from build123d import *

# Parameters (mm, degrees)
BOSS_EXTRU_1_DEPTH      = 30
ESQUISSE2_R             = 15
BOSS_EXTRU_2_DEPTH      = 5
BOSS_EXTRU_3_DEPTH      = 10
ESQUISSE7_R             = 2
ENL_V_MAT_EXTRU_1_DEPTH = 10


with BuildPart() as part:
    # Esquisse1 → Boss.-Extru.1 (new body)
    with BuildSketch(Plane.XY):
        Polygon((-14.849242405, 0), (0, 14.849242405), (14.849242405, 0), (19.849242405, 0), (0, 19.849242405), (-19.849242405, 0), align=None)
    extrude(amount=BOSS_EXTRU_1_DEPTH)

    # Esquisse2 → Boss.-Extru.2 (add)
    with BuildSketch(Plane(origin=(0, 14.849242405, 0), x_dir=(1, 0, 0), z_dir=(0, 1, 0))):
        with Locations((0, -15)):
            Circle(ESQUISSE2_R)
    extrude(amount=BOSS_EXTRU_2_DEPTH)

    # Esquisse5 → Boss.-Extru.3 (add)
    with BuildSketch(Plane(origin=(0, 19.849242405, 0), x_dir=(1, 0, 0), z_dir=(0, 1, 0))):
        with BuildLine():
            ThreePointArc((5, -9.409830056), (0, -7.5), (-5, -9.409830056))
            Line((-5, -9.409830056), (-5, -15))
            Line((-5, -15), (5, -15))
            Line((5, -15), (5, -9.409830056))
        make_face()
        with BuildLine():
            Line((5, -15), (-5, -15))
            Line((-5, -15), (-5, -20.590169944))
            ThreePointArc((-5, -20.590169944), (0, -22.5), (5, -20.590169944))
            Line((5, -20.590169944), (5, -15))
        make_face()
    extrude(amount=BOSS_EXTRU_3_DEPTH)

    # Esquisse7 → Enlèv. mat.-Extru.1 (cut)
    with BuildSketch(Plane.ZY.offset(5)):
        with Locations((15, 24.849242405)):
            Circle(ESQUISSE7_R)
    extrude(amount=-ENL_V_MAT_EXTRU_1_DEPTH, mode=Mode.SUBTRACT)


solid = part.part
Here's how the part is built. I have some questions about the finished solid (model axes, mm). A direction names the side the tool comes from. Give positions to 0.01 mm unless a question says otherwise; leave off trailing zeros. Order: outer loops, then holes, each group sorted by start corner. A loop starts at its lowest first (then second) coordinate and runs counter-clockwise, first axis right, second up. Notation, with made-up numbers: (-16, -29.75) -> (-6, -29.75) arc R20 ccw to (-6, 0.25) -> close; hole circle Ø5 at (15.25, 15.5). An arc over 180 degrees is marked (long way). Use a Markdown table: item, result. Add a question column.
Item 1: I need wall thicknesses on line 1 (Y direction, x = -13, z = 17.5); line 2 (Z direction, x = -2.5, y = 24.25); line 3 (X direction, y = 7.5, z = 17). Which ranges of each line are inside material? Lowest first, please.
Item 2: Imagine slicing it at D-D on x = 4. Please give me the cut outline in (y, z).
Item 3: Imagine slicing it at A-A on z = 15. Please give me the cut outline in (x, y).
Item 4: If we mould it in two halves opening along Y, with no side actions, what happens to faces 4 (the face through (0.1, 24.8, 7.5)), 5 (the face through (-11.99, 7.86, 14.79)), 6 (the face through (-17, 0, 15))? For each: pulls with the +Y half, pulls with the -Y half, needs draft (parallel to the pull), parting line crosses it, or undercut.
Item 5: Imagine slicing it at C-C on x = -5.5. Please give me the cut outline in (y, z).
Item 6: For faces 1 (the face through (-15, 17, 15)), 2 (the face through (5, 22.6, 15.1)), 3 (the face through (-5, 22.6, 14.9)), which set-ups out of +Z, -Z, +X, -X, +Y, -Y let a thin tool reach every point of the face, with its end or its side?
Item 7: Will these pins go through, and if not, where does the flat tip stop? pin 1 (5 mm diameter, centred on x = 0, y = 26, fed in from -Z); pin 2 (2 mm diameter, centred on y = 12, z = 20, fed in from -X); pin 3 (11 mm diameter, centred on x = 8, z = 9.5, fed in from -Y); pin 4 (2 mm diameter, centred on x = -6.5, y = 25.5, fed in from +Z).
Item 8: Imagine slicing it at B-B on y = 13. Please give me the cut outline in (x, z).
Data:
| question | item | result |
|---|---|---|
| 1 | line 1 | y = 1.85 to 6.85, 14.85 to 19.85 |
| 1 | line 2 | z = 7.93 to 13.09, 16.91 to 22.07 |
| 1 | line 3 | x = -12.35 to -7.35, 7.35 to 12.35 |
| 2 | outline | (10.85, 0) -> (15.85, 0) -> (15.85, 0.54) -> (19.85, 0.54) -> (19.85, 8.66) -> (29.85, 8.66) -> (29.85, 21.34) -> (19.85, 21.34) -> (19.85, 29.46) -> (15.85, 29.46) -> (15.85, 30) -> (10.85, 30) -> close; hole circle Ø4 at (24.85, 15) |
| 3 | outline | (-19.85, 0) -> (-14.85, 0) -> (0, 14.85) -> (14.85, 0) -> (19.85, 0) -> (5, 14.85) -> (15, 14.85) -> (15, 19.85) -> (5, 19.85) -> (5, 22.85) -> (-5, 22.85) -> (-5, 19.85) -> (-15, 19.85) -> (-15, 14.85) -> (-5, 14.85) -> close; (-5, 26.85) -> (5, 26.85) -> (5, 29.85) -> (-5, 29.85) -> close |
| 4 | face 4 | needs draft |
| 4 | face 5 | undercut |
| 4 | face 6 | pulls with the -Y half |
| 5 | outline | (9.35, 0) -> (14.35, 0) -> (14.35, 30) -> (9.35, 30) -> close; (14.85, 1.04) -> (19.85, 1.04) -> (19.85, 28.96) -> (14.85, 28.96) -> close |
| 6 | face 1 | -X, +Y |
| 6 | face 2 | +Z, -Z, +X, +Y |
| 6 | face 3 | +Z, -Z, -X, +Y |
| 7 | pin 1 | stops at z = 7.5 |
| 7 | pin 2 | stops at x = -8.85 |
| 7 | pin 3 | stops at y = 1.35 |
| 7 | pin 4 | passes through |
| 8 | outline | (-6.85, 0) -> (-1.85, 0) -> (-1.85, 30) -> (-6.85, 30) -> close; (1.85, 0) -> (6.85, 0) -> (6.85, 30) -> (1.85, 30) -> close |
